Part model, mm, in its own coordinate system. A direction names the side the tool comes from. Coordinates: 2 decimals unless noted, no trailing zeros. Order: outer loops, then holes, each group sorted by start corner. A loop starts at its lowest first (then second) coordinate and runs counter-clockwise, first axis right, second up.
from build123d import *

# Parameters (mm, degrees)
SALIENTE_EXTRUIR1_DEPTH = 7.5
SALIENTE_EXTRUIR2_DEPTH = 7.5
CROQUIS3_R              = 2.25
CORTAR_EXTRUIR1_DEPTH   = 45.240818256
CROQUIS4_R              = 4
CORTAR_EXTRUIR2_DEPTH   = 41.959224846
CORTAR_EXTRUIR3_DEPTH   = 3.5
CORTAR_EXTRUIR4_DEPTH   = 15
SIMETR_A3_COPY_1_DEPTH  = 3.5


with BuildPart() as part:
    # Croquis1 → Saliente-Extruir1 (new, symmetric)
    with BuildSketch(Plane.XY):
        with BuildLine():
            Line((-26, 0), (-21, 0))
            ThreePointArc((-21, 0), (0, 21), (21, 0))
            Line((21, 0), (26, 0))
            ThreePointArc((26, 0), (0, 26), (-26, 0))
        make_face()
    extrude(amount=SALIENTE_EXTRUIR1_DEPTH, both=True)

    # Croquis2 → Saliente-Extruir2 (add, symmetric)
    with BuildSketch(Plane.XY):
        with BuildLine():
            Line((26, 0), (35, 0))
            Line((35, 0), (35, 5))
            Line((35, 5), (21.236760582, 15))
            ThreePointArc((21.236760582, 15), (24.78059498, 7.869060455), (26, 0))
        make_face()
    saliente_extruir2 = extrude(amount=SALIENTE_EXTRUIR2_DEPTH, both=True)

    # Croquis3 → Cortar-Extruir1 (cut, through all)
    with BuildSketch(Plane.XZ):
        with Locations(Location((31, 0, 0), (0, 0, 270))):
            Circle(CROQUIS3_R)
    cortar_extruir1 = extrude(amount=-CORTAR_EXTRUIR1_DEPTH, mode=Mode.SUBTRACT)

    # Croquis4 → Cortar-Extruir2 (cut, through all)
    with BuildSketch(Plane(origin=(0, 6.09, 0), x_dir=(-1, 0, 0), z_dir=(0, -1, 0))):
        with Locations((-31, 0)):
            Circle(CROQUIS4_R)
    cortar_extruir2 = extrude(amount=-CORTAR_EXTRUIR2_DEPTH, mode=Mode.SUBTRACT)

    # Simetría1: Saliente-Extruir2, Cortar-Extruir1, Cortar-Extruir2 across plane
    add(saliente_extruir2.mirror(Plane(origin=(0, 0, 0), x_dir=(0, 0, 1), z_dir=(1, 0, 0))))
    add(cortar_extruir1.mirror(Plane(origin=(0, 0, 0), x_dir=(0, 0, 1), z_dir=(1, 0, 0))), mode=Mode.SUBTRACT)
    add(cortar_extruir2.mirror(Plane(origin=(0, 0, 0), x_dir=(0, 0, 1), z_dir=(1, 0, 0))), mode=Mode.SUBTRACT)

    # Croquis6 → Cortar-Extruir3 (cut)
    with BuildSketch(Plane.XY.offset(7.5)):
        with BuildLine():
            Line((31.403995152, 3.90450261), (22.755647062, 10.188159987))
            ThreePointArc((22.755647062, 10.188159987), (22.148664364, 10.17350309), (22.003343347, 9.5839909))
            ThreePointArc((22.003343347, 9.5839909), (23.084675568, 6.564887959), (23.753839647, 3.428571429))
            ThreePointArc((23.753839647, 3.428571429), (23.921384471, 3.122035527), (24.248711306, 3))
            Line((24.248711306, 3), (31.110094423, 3))
            ThreePointArc((31.110094423, 3), (31.585621134, 3.34548674), (31.403995152, 3.90450261))
        make_face()
    cortar_extruir3 = extrude(amount=-CORTAR_EXTRUIR3_DEPTH, mode=Mode.SUBTRACT)

    # Simetría2: Cortar-Extruir3 across plane
    add(cortar_extruir3.mirror(Plane.XY), mode=Mode.SUBTRACT)

    # Croquis8 → Cortar-Extruir4 (cut)
    with BuildSketch(Plane(origin=(0, 26, 0), x_dir=(1, 0, 0), z_dir=(0, 1, 0))):
        with BuildLine():
            Line((-16.736760582, -4.5), (16.736760582, -4.5))
            ThreePointArc((16.736760582, -4.5), (17.797420753, -4.060660172), (18.236760582, -3))
            Line((18.236760582, -3), (18.236760582, 3))
            ThreePointArc((18.236760582, 3), (17.797420753, 4.060660172), (16.736760582, 4.5))
            Line((16.736760582, 4.5), (-16.736760582, 4.5))
            ThreePointArc((-16.736760582, 4.5), (-17.797420753, 4.060660172), (-18.236760582, 3))
            Line((-18.236760582, 3), (-18.236760582, -3))
            ThreePointArc((-18.236760582, -3), (-17.797420753, -4.060660172), (-16.736760582, -4.5))
        make_face()
    extrude(amount=-CORTAR_EXTRUIR4_DEPTH, mode=Mode.SUBTRACT)

    # Simetría3: Cortar-Extruir3 across plane
    add(cortar_extruir3.mirror(Plane(origin=(0, 0, 0), x_dir=(0, 0, 1), z_dir=(1, 0, 0))), mode=Mode.SUBTRACT)

    # Simetría3 copy 1 sketch → Simetría3 copy 1 (cut)
    with BuildSketch(Plane(origin=(0, 0, -7.5), x_dir=(-1, 0, 0), z_dir=(0, 0, -1))):
        with BuildLine():
            Line((31.403995152, 3.90450261), (22.755647062, 10.188159987))
            ThreePointArc((22.755647062, 10.188159987), (22.148664364, 10.17350309), (22.003343347, 9.5839909))
            ThreePointArc((22.003343347, 9.5839909), (23.084675568, 6.564887959), (23.753839647, 3.428571429))
            ThreePointArc((23.753839647, 3.428571429), (23.921384471, 3.122035527), (24.248711306, 3))
            Line((24.248711306, 3), (31.110094423, 3))
            ThreePointArc((31.110094423, 3), (31.585621134, 3.34548674), (31.403995152, 3.90450261))
        make_face()
    extrude(amount=-SIMETR_A3_COPY_1_DEPTH, mode=Mode.SUBTRACT)


solid = part.part
Q1. Cut at C-C on x = -1. Write the cut outline in (y, z).
Results list:
outline: (20.98, -7.5) - (25.98, -7.5) - (25.98, -4.5) - (20.98, -4.5) - close; (20.98, 4.5) - (25.98, 4.5) - (25.98, 7.5) - (20.98, 7.5) - close
Q2. Wall check: line 1 along Z through (x, y) = (12.5, 18); line 2 along X through (y, z) = (8.75, 5); line 3 along Z through (x, y) = (-31, 2.75). Give the ranges that are in metal, low to high.
Results list:
line 1: z = -7.5 to -4.5, 4.5 to 7.5
line 2: x = -29.84 to -24.74, -22.35 to -19.09, 19.09 to 22.35, 24.74 to 29.84
line 3: z = -7.5 to -2.25, 2.25 to 7.5
Q3. Cut at D-D on y = 7. Write the cut outline in (x, z).
Results list:
outline: (-32.25, -7.5) - (-27.14, -7.5) - (-27.14, -4) - (-22.96, -4) - (-22.96, -7.5) - (-19.8, -7.5) - (-19.8, 7.5) - (-22.96, 7.5) - (-22.96, 4) - (-27.14, 4) - (-27.14, 7.5) - (-32.25, 7.5) - (-32.25, 3.8) arc R4 cw (long way) to (-32.25, -3.8) - close; (19.8, -7.5) - (22.96, -7.5) - (22.96, -4) - (27.14, -4) - (27.14, -7.5) - (32.25, -7.5) - (32.25, -3.8) arc R4 cw (long way) to (32.25, 3.8) - (32.25, 7.5) - (27.14, 7.5) - (27.14, 4) - (22.96, 4) - (22.96, 7.5) - (19.8, 7.5) - close
Q4. Mould opens along X. For faces 5 (the face through (-26.69, 11.04, 0.11)), 6 (the face through (28, 3, -6)), 7 (the face through (0, 22, -7.5)) say: pulls with the +X half, pulls with the -X half, needs draft (parallel to the pull), parting line crosses it, or undercut.
Results list:
face 5: pulls with the -X half
face 6: undercut
face 7: needs draft
Q5. Pin check, flat tips, straight feed: pin 1 Ø3 at (y, z) = (12.5, -6) entering from -X; pin 2 Ø4 at (x, z) = (26.5, 5) entering from +Y; pin 3 Ø1 at (x, z) = (1, -4.5) entering from -Y; pin 4 Ø6.5 at (x, y) = (2, 18) entering from -Z. Stop position of each tip, or through.
Results list:
pin 1: stops at x = -26.74
pin 2: stops at y = 12.63
pin 3: stops at y = 20.95
pin 4: stops at z = -7.5
Q6. Cut at A-A on z = 0. Write the cut outline in (x, y).
Results list:
outline: (-35, 0) - (-33.25, 0) - (-33.25, 6.09) - (-33.5, 6.09) - (-35, 5) - close; (-28.75, 0) - (-21, 0) arc R21 cw to (-17.89, 11) - (-18.24, 11) - (-18.24, 18.53) arc R26 ccw to (-21.24, 15) - (-27, 10.81) - (-27, 6.09) - (-28.75, 6.09) - close; (17.89, 11) arc R21 cw to (21, 0) - (28.75, 0) - (28.75, 6.09) - (27, 6.09) - (27, 10.81) - (21.24, 15) arc R26 ccw to (18.24, 18.53) - (18.24, 11) - close; (33.25, 0) - (35, 0) - (35, 5) - (33.5, 6.09) - (33.25, 6.09) - close
Q7. Cut at B-B on y = 22.25. Write the cut outline in (x, z), and give its area (3 significant figures).
Results list:
outline: (-13.45, -7.5) - (13.45, -7.5) - (13.45, -4.5) - (-13.45, -4.5) - close; (-13.45, 4.5) - (13.45, 4.5) - (13.45, 7.5) - (-13.45, 7.5) - close
area: 161 mm2
Q8. Which spindle directions (+Z, -Z, +X, -X, +Y, -Y) get a long thin tool onto all of the face, cutting with end or side? Do faces 1 (the face through (-26, 6, -4)), 2 (the face through (28, 3, 6)), 3 (the face through (27, 8, 0)), 4 (the face through (-28, 0, 0)). Say none if no direction does.
Results list:
face 1: -Z
face 2: +Z
face 3: +Y
face 4: +Z, -Z, +X, -X, -Y
